from build123d import *

# Parameters (mm, degrees)
SKETCH1_R           = 6.54812
BOSS_EXTRUDE3_DEPTH = 6.35


with BuildPart() as part:
    # Sketch1 → Boss-Extrude3 (new body)
    with BuildSketch(Plane(origin=(0, 0, 0), x_dir=(1, 0, 0), z_dir=(0, 1, 0))):
        with BuildLine():
            Line((-19.473738898, 31.474503951), (-19.473738898, -18.151447985))
            Line((-19.473738898, -18.151447985), (5.926261102, -18.151447985))
            Line((5.926261102, -18.151447985), (5.926261102, 31.474503951))
            ThreePointArc((5.926261102, 31.474503951), (-6.773738898, 45.402703843), (-19.473738898, 31.474503951))
        make_face()
        with Locations(Location((-6.773738898, 32.648552015, 0), (0, 0, 270))):
            Circle(SKETCH1_R, mode=Mode.SUBTRACT)
    extrude(amount=-BOSS_EXTRUDE3_DEPTH)


solid = part.part
Verification items for the finished model (mm, model axes). A direction names the side the tool comes from. Round coordinates to 2 decimals unless told otherwise and drop trailing zeros. Loops run counter-clockwise (first coordinate to the right, second up) from the corner with the lowest first, then second, coordinate; pieces in that order, holes last. Notation, with made-up numbers: (77.25, -31.75) - (85.25, -31.75) arc R28 ccw to (85.25, 4.25) - close; hole circle Ø3 at (-7, -29.5). An arc over 180 degrees is marked (long way). Write item = value, one per line.
Q1. Material ranges on L1, parallel to X at y = -5, z = 15.5; L2, parallel to X at y = -1.5, z = -38; L3, parallel to Z at x = -2.75, y = -1.75, recorded low to high.
Here are the results:
L1 = -19.47 to 5.93
L2 = -18.35 to -10.55, -3 to 4.8
L3 = -44.75 to -37.81, -27.48 to 18.15
Q2. Depth check by flat-ended pin: pin 1 (4 mm diameter, centred on x = -2.5, z = -37.5, fed in from +Y); pin 2 (10.5 mm diameter, centred on x = -6.77, z = -32.65, fed in from +Y); pin 3 (3 mm diameter, centred on y = -3.5, z = -1, fed in from +X). Enter the tip coordinate at first touch or a pass-through.
Here are the results:
pin_1 = 0
pin_2 = through
pin_3 = 5.93
Q3. Sectioned sample at D-D on x = -14.25. Record the boundary of the cut face in (y, z), plus the area to 3 significant figures.
Here are the results:
outline = (-6.35, -42.98) - (0, -42.98) - (0, 18.15) - (-6.35, 18.15) - close
area = 388 mm^2
Q4. Sectioned sample at A-A on x = -4. Record the boundary of the cut face in (y, z), plus the area to 3 significant figures.
Here are the results:
outline = (-6.35, -45.1) - (0, -45.1) - (0, -38.58) - (-6.35, -38.58) - close; (-6.35, -26.72) - (0, -26.72) - (0, 18.15) - (-6.35, 18.15) - close
area = 326 mm^2
Q5. Mould release check, pull along X, two halves, no side actions. Record for faces 1 (the flat face through (-7, -3, 18.151)), 2 (the flat face through (-19.474, -3, -7)), 3 (the cylindrical face through (-4.81, -3.13, -26.4)), 4 (the cylindrical face through (-6.5, -3.1, -45.4)): +X half, -X half, draft (parallel to the pull), parting line (faces both ways), or undercut.
Here are the results:
face_1 = draft
face_2 = -X half
face_3 = undercut
face_4 = parting line
Q6. Tool access check on faces 5 (the flat face through (5.926, -3, -6)), 6 (the flat face through (-7, -6.35, -7)). Record the directions out of +Z, -Z, +X, -X, +Y, -Y that give a thin tool (end or side, any length) a straight path to the whole face; none if there is none.
Here are the results:
face_5 = +Z, +X, +Y, -Y
face_6 = +Z, -Z, +X, -X, -Y
Q7. Sectioned sample at C-C on y = -4.75. Record the boundary of the cut face in (x, z).
Here are the results:
outline = (-19.47, -31.47) arc R12.75 ccw (long way) to (5.93, -31.47) - (5.93, 18.15) - (-19.47, 18.15) - close; hole circle Ø13.1 at (-6.77, -32.65)
Q8. Sectioned sample at B-B on z = -36. Record the boundary of the cut face in (x, y), plus the area to 3 significant figures.
Here are the results:
outline = (-19.08, -6.35) - (-12.4, -6.35) - (-12.4, 0) - (-19.08, 0) - close; (-1.15, -6.35) - (5.53, -6.35) - (5.53, 0) - (-1.15, 0) - close
area = 84.8 mm^2
